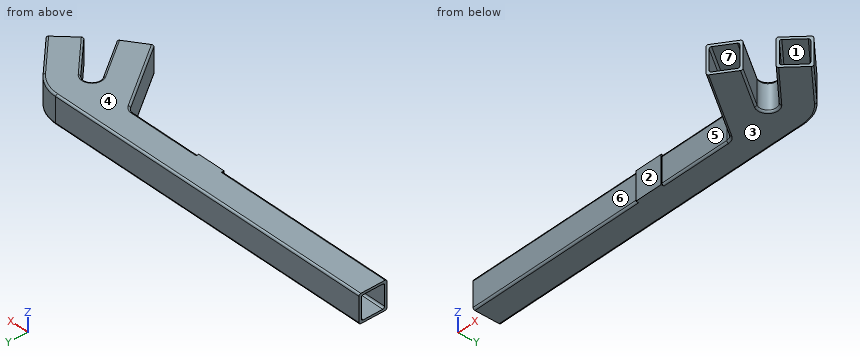
Autodesk Inventor part; units mm, degrees
ref_plane "YZ Plane" through (0, 0, 0) normal (1, 0, 0) x (0, 1, 0)
ref_plane "XZ Plane" through (0, 0, 0) normal (0, 1, 0) x (-1, 0, 0)
ref_plane "XY Plane" through (0, 0, 0) normal (0, 0, 1) x (1, 0, 0)
sketch "Sketch1" plane through (0, 0, 0) normal (0, 0, 1) x (1, 0, 0)
  line L0 (98.7752, 71.1622) -> (146.7319, 2.6729)
  line L1 (146.7319, 2.6729) -> (171.3065, 19.8802)
  line L2 (171.3065, 19.8802) -> (142.6276, 60.8378)
  arc A0 (156.364, 72.364) -> (142.6276, 60.8378) centre (150, 66) ccw
  line L3 (156.364, 72.364) -> (191.7193, 37.0086)
  line L4 (191.7193, 37.0086) -> (212.9325, 58.2218)
  line L5 (212.9325, 58.2218) -> (177.5772, 93.5772)
  arc A1 (177.5772, 93.5772) -> (150, 105) centre (150, 66) ccw
  line L6 (91.4028, 75) -> (-208.5972, 75)
  line L7 (150, 105) -> (-208.5972, 105)
  line L8 (-208.5972, 105) -> (-208.5972, 75)
  line L9 (0, 128.7567) -> (0, -18.341)
  line L10 (-292.9031, 0) -> (297.2384, 0)
  arc A2 (98.7752, 71.1622) -> (91.4028, 75) centre (91.4028, 66) ccw
  dimension "d38" = 30
  dimension "d39" = 30
  dimension "d40" = 9
  dimension "d47" = 30
  dimension "d53" = 9
  dimension "d56" = 300
  dimension "d58" = 150
  dimension "d59" = 50
  dimension "d60" = 35
  dimension "d61" = 75
  dimension "d88" = 45
extrude "Extrusion1" add sketch "Sketch1" along normal mid plane 30
sketch "Sketch4" plane through (0, 0, 0) normal (0, 0, 1) x (1, 0, 0)
  line L0 (-208.5972, 75) -> (91.4028, 75)
  line L1 (-15, 75) -> (15, 75)
  line L2 (-15, 75) -> (-15, 74)
  line L3 (-15, 74) -> (15, 74)
  line L4 (15, 74) -> (15, 75)
  line L5 (0, 90) -> (0, -15)
  point P0 (0, 0)
  dimension "d62" = 30
  dimension "d63" = 15
  dimension "d64" = 1
extrude "Extrusion4" add sketch "Sketch4" along normal mid plane 30
fillet "Fillet1" radius 2 14 edges at (-111.7986, 75, 15) (95.5586, 73.9831, 15) (122.7535, 36.9176, 15) (53.2014, 75, 15) (-111.7986, 75, -15) (95.5586, 73.9831, -15) (122.7535, 36.9176, -15) (53.2014, 75, -15) (164.9247, 102.0313, -15) (195.2548, 75.8995, -15) (-29.2986, 105, -15) (164.9247, 102.0313, 15) (195.2548, 75.8995, 15) (-29.2986, 105, 15)
sketch "Sketch5" plane through (-208.5972, 77, -15) normal (-1, 0, 0) x (0, 0, 1)
  line L0 (27.5, 25.5) -> (2.5, 25.5)
  line L1 (2.5, 25.5) -> (2.5, 0.5)
  line L2 (2.5, 0.5) -> (27.5, 0.5)
  line L3 (27.5, 0.5) -> (27.5, 25.5)
  line L4 (2, 28) -> (28, 28)
  line L5 (0, 0) -> (0, 26)
  line L6 (2, -2) -> (28, -2)
  line L7 (30, 26) -> (30, 0)
  point P0 (15, -77)
  dimension "d68" = 2.5
  dimension "d69" = 2.5
  dimension "d70" = 2.5
  dimension "d71" = 2.5
extrude "Extrusion5" cut sketch "Sketch5" against normal blind 350
fillet "Fillet2" radius 2 4 edges at (-33.5972, 77.5, 12.5) (-33.5972, 77.5, -12.5) (-33.5972, 102.5, -12.5) (-33.5972, 102.5, 12.5)
sketch "Sketch6" plane through (191.7193, 37.0086, -15) normal (0.7071, -0.7071, 0) x (0.7071, 0.7071, 0)
  line L0 (2.5, 27.5) -> (27.5, 27.5)
  line L1 (27.5, 27.5) -> (27.5, 2.5)
  line L2 (27.5, 2.5) -> (2.5, 2.5)
  line L3 (2.5, 2.5) -> (2.5, 27.5)
  line L4 (28, 0) -> (0, 0)
  line L5 (30, 2) -> (30, 28)
  line L6 (0, 30) -> (28, 30)
  line L7 (0, 0) -> (0, 30)
  point P0 (-161.7351, 15)
  dimension "d75" = 2.5
  dimension "d76" = 2.5
  dimension "d77" = 2.5
  dimension "d78" = 2.5
extrude "Extrusion6" cut sketch "Sketch6" against normal blind 50
sketch "Sketch7" plane through (171.3065, 19.8802, -15) normal (0.5736, -0.8192, 0) x (0.8192, 0.5736, 0)
  line L0 (-27.5, 27.5) -> (-2.5, 27.5)
  line L1 (-2.5, 27.5) -> (-2.5, 2.5)
  line L2 (-2.5, 2.5) -> (-27.5, 2.5)
  line L3 (-27.5, 2.5) -> (-27.5, 27.5)
  line L4 (-28, 30) -> (0, 30)
  line L5 (0, 30) -> (0, 0)
  line L6 (0, 0) -> (-28, 0)
  line L7 (-30, 2) -> (-30, 28)
  point P0 (-151.7289, 15)
  dimension "d81" = 2.5
  dimension "d82" = 2.5
  dimension "d83" = 2.5
  dimension "d84" = 2.5
extrude "Extrusion7" cut sketch "Sketch7" against normal blind 50
fillet "Fillet3" radius 2 14 edges at (174.0416, 54.6863, 15) (156.967, 40.359, 15) (144.2149, 72.8944, 15) (156.967, 40.359, -15) (174.0416, 54.6863, -15) (144.2149, 72.8944, -15) (134.4404, 24.5857, -12.5) (134.4404, 24.5857, 12.5) (154.9192, 38.9251, 12.5) (154.9192, 38.9251, -12.5) (175.8094, 56.4541, -12.5) (193.4871, 74.1317, -12.5) (193.4871, 74.1317, 12.5) (175.8094, 56.4541, 12.5)
equation "\"d39\" = d38"
equation "\"secure_arm_radii\" = 9"
equation "\"rack_tooth_thickness\" = 5"
equation "\"rack_tooth_addendum\" = 5"
equation "\"rack_tooth_dedendum\" = 5"
equation "\"hoop_width_large\" = 51"
equation "\"hoop_thickness_large\" = 4"
equation "\"hoop_width_medium\" = 33.7"
equation "\"hoop_thickness_medium\" = 3.2"
equation "\"hoop_width_small\" = 25.4"
equation "\"hoop_thickness_small\" = 2"
equation "\"hoop_bearing_length\" = 5deg"
equation "\"secure_arm_angle\" = 35deg"
equation "\"hoop_tabs_thickness\" = 6"
equation "\"hoop_tabs_hole\" = 12"
equation "\"support_baseClamp_thickness\" = 8"
equation "\"support_frame_endHoleBuffer\" = 45"
equation "\"support_frame_squareBarThickness\" = 5"
equation "\"support_baseClamp_sleeveSweepTerminationAngle\" = 55deg"
equation "\"support_baseClamp_sleeveHoleDiameter\" = 12"
equation "\"support_frame_squareBarFillet\" = 2"
equation "\"support_baseClamp_platformWidthBuffer\" = 0"
equation "\"support_baseClamp_platformThickness\" = 15"
equation "\"support_baseClamp_platformLengthBuffer\" = 35"
equation "\"hoop_angle_z\" = 45deg"
equation "\"hoop_cable_diam\" = 5"
equation "\"hoop_cable_pulley_diam\" = 22"
equation "\"wheelchair_deployed_width\" = 635"
equation "\"wheelchair_deployed_height\" = 914"
equation "\"wheelchair_deployed_length\" = 1067"
equation "\"sm_varx_pinPlate_thickness\" = 5"
equation "\"sm_varx_member_tolerance\" = 0"
equation "\"sm_varx_pinPlate_holeDiameter\" = 5"
equation "\"sm_varx_squareBarThickness\" = 2.5"
equation "\"hoop_bushing23_radialInterference\" = 0"
equation "\"hoop_bushing12_radialInterference\" = 0"
equation "\"hoop_bushing12_od\" = 43"
equation "\"hoop_bushing23_od\" = 27.3"
equation "\"wheelchatir_pos_deploy_angle_0\" = 65deg"
equation "\"wheelchatir_pos_store_angle_0\" = 90deg"
equation "\"wheelchatir_pos_deploy_angle_1\" = 20deg"
equation "\"wheelchatir_pos_store_angle_1\" = 20deg"
equation "\"hoop_bushing12_thickness\" = 9.3"
equation "\"hoop_bushing23_thickness\" = 1.9"
properties part number "grip_N_fix"
The model under review builds one solid part; all positions refer to its coordinate system, in mm. Face numbers are marked on the shaded views. A direction names the side the tool comes from. Round coordinates to 2 decimals unless told otherwise and drop trailing zeros. Loops run counter-clockwise (first coordinate to the right, second up) from the corner with the lowest first, then second, coordinate; pieces in that order, holes last. Notation, with made-up numbers: (45, -30) -> (84, -30) arc R31 cw to (84, 1) -> close; hole circle Ø6 at (-29.75, -5). An arc over 180 degrees is marked (long way). Write item = value, one per line. Start each with the question number.
Item 1: Take a section at C-C on x = -114. Give the boundary of the cut face in (y, z), plus the area to 3 significant figures.
Item 2: Take a section at B-B on z = -6. Give the boundary of the cut face in (x, y), plus the area to 3 significant figures.
Item 3: Take a section at A-A on x = 7. Give the boundary of the cut face in (y, z).
Item 4: Mouldability with a two-part tool opening along X and no side actions: class the marked faces 6 and 7 as released by +X, released by -X, zero draft, split by the parting line, or undercut.
Item 5: To check wall thickness, follow L1, parallel to Y at x = -147, z = -6; L2, parallel to Y at x = 29, z = 11; L3, parallel to Z at x = -161.5, y = 96.5. State the ranges of each line that lie inside material, in increasing order.
Item 6: For the marked faces 1, 2, 3, 4 and 5, list the 3-axis set-ups (+Z, -Z, +X, -X, +Y, -Y) from which the entire face can be reached by the end or side of a thin tool; tool diameter is ignored.
Item 7: Insertion check: pin 1 (7.5 mm diameter, centred on y = 90, z = -1.5, fed in from -X); pin 2 (8 mm diameter, centred on x = -28.5, z = -7, fed in from -Y); pin 3 (4 mm diameter, centred on x = 131, z = -2, fed in from -Y). Each pin has a flat end and moves straight along its axis. Give the tip position at first contact, or say it passes through.
Result:
q1.outline = (75, -13) arc R2 ccw to (77, -15) -> (103, -15) arc R2 ccw to (105, -13) -> (105, 13) arc R2 ccw to (103, 15) -> (77, 15) arc R2 ccw to (75, 13) -> close; hole (77.5, -10.5) arc R2 ccw to (79.5, -12.5) -> (100.5, -12.5) arc R2 ccw to (102.5, -10.5) -> (102.5, 10.5) arc R2 ccw to (100.5, 12.5) -> (79.5, 12.5) arc R2 ccw to (77.5, 10.5) -> close
q1.area = 275 mm²
q2.outline = (-208.6, 75) -> (-15, 75) -> (-15, 74) -> (15, 74) -> (15, 75) -> (91.4, 75) arc R9 cw to (98.78, 71.16) -> (146.73, 2.67) -> (148.78, 4.11) -> (120.1, 45.07) -> (140.58, 59.41) -> (169.26, 18.45) -> (171.31, 19.88) -> (142.63, 60.84) arc R9 cw to (156.36, 72.36) -> (191.72, 37.01) -> (193.49, 38.78) -> (158.13, 74.13) -> (175.81, 91.81) -> (211.16, 56.45) -> (212.93, 58.22) -> (177.58, 93.58) arc R39 ccw to (150, 105) -> (-208.6, 105) -> (-208.6, 102.5) -> (141.4, 102.5) -> (141.4, 77.5) -> (-208.6, 77.5) -> close
q2.area = 4,010 mm²
q3.outline = (74, -15) -> (103, -15) arc R2 ccw to (105, -13) -> (105, 13) arc R2 ccw to (103, 15) -> (74, 15) -> close; hole (77.5, -10.5) arc R2 ccw to (79.5, -12.5) -> (100.5, -12.5) arc R2 ccw to (102.5, -10.5) -> (102.5, 10.5) arc R2 ccw to (100.5, 12.5) -> (79.5, 12.5) arc R2 ccw to (77.5, 10.5) -> close
q4.face_6 = zero draft
q4.face_7 = undercut
q5.L1 = 75 to 77.5, 102.5 to 105
q5.L2 = 75 to 77.56, 102.44 to 105
q5.L3 = -15 to -12.5, 12.5 to 15
q6.face_1 = none
q6.face_2 = +Z, -Z, -X, -Y
q6.face_3 = -Z, +X, -X, +Y, -Y
q6.face_4 = +Z, +X, -X, +Y, -Y
q6.face_5 = +Z, -Z, -Y
q7.pin_1 = 141.4
q7.pin_2 = 75
q7.pin_3 = 22.28
